```python
from build123d import *

# Parameters (mm, degrees)
SKETCH_1_W      = 5
SKETCH_1_H      = 7
SKETCH_1_H_2    = 14
SKETCH_1_W_2    = 30
SKETCH_1_H_3    = 5
EXTRUDE_2_DEPTH = 5


with BuildPart() as part:
    # 草图1 → 凸台-拉伸2 (new body)
    with BuildSketch(Plane.XY):
        with Locations((-106.5, 21.5)):
            Rectangle(SKETCH_1_W, SKETCH_1_H)
        with Locations((-111.5, 18)):
            Rectangle(SKETCH_1_W, SKETCH_1_H_2)
        Polygon((-64, 0), (-54, 0), (-54, 7), (-55.5, 7), (-55.5, 9.9), (-54, 9.9), (-54, 11), (-52, 11), (-52, 25), (-104, 25), (-104, 18), (-104, 0), (-94, 0), align=None)
        Polygon((-50, 7), (-50, 0), (-40, 0), (-10, 0), (0, 0), (0, 18), (0, 25), (-52, 25), (-52, 11), (-50, 11), (-50, 9.9), (-48.5, 9.9), (-48.5, 7), align=None)
        with Locations((7.5, 18)):
            Rectangle(SKETCH_1_W, SKETCH_1_H_2)
        with Locations((2.5, 21.5)):
            Rectangle(SKETCH_1_W, SKETCH_1_H)
        with Locations((-25, -2.5)):
            Rectangle(SKETCH_1_W_2, SKETCH_1_H_3)
        with Locations((-79, -2.5)):
            Rectangle(SKETCH_1_W_2, SKETCH_1_H_3)
    extrude(amount=EXTRUDE_2_DEPTH)


solid = part.part
```
Part model, mm, in its own coordinate system. A direction names the side the tool comes from. Round coordinates to 2 decimals unless told otherwise and drop trailing zeros. Write each loop counter-clockwise with the first axis right and the second up, starting at its lowest first coordinate (ties: lowest second). Pieces come first, ordered by that corner, then holes.
Item 1: Cut at A-A, the plane y = -3. Give the cut face in (x, z), plus the area to 3 significant figures.
Results:
outline: (-94, 0) - (-64, 0) - (-64, 5) - (-94, 5) - close; (-40, 0) - (-10, 0) - (-10, 5) - (-40, 5) - close
area: 300 mm2
Item 2: Probe L1, parallel to X at y = 16.25, z = 0.35; L2, parallel to X at y = -1.5, z = 4.45; L3, parallel to X at y = 8.25, z = 1.4. List the from-to ranges inside material, lowest first.
Results:
L1: x = -114 to -109, -104 to 0, 5 to 10
L2: x = -94 to -64, -40 to -10
L3: x = -104 to -55.5, -48.5 to 0
Item 3: Cut at B-B, the plane y = 12.25. Give the cut face in (x, z), plus the area to 3 significant figures.
Results:
outline: (-114, 0) - (-109, 0) - (-109, 5) - (-114, 5) - close; (-104, 0) - (0, 0) - (0, 5) - (-104, 5) - close; (5, 0) - (10, 0) - (10, 5) - (5, 5) - close
area: 570 mm2
Item 4: Cut at D-D, the plane y = 3.75. Give the cut face in (x, z), plus the area to 3 significant figures.
Results:
outline: (-104, 0) - (-54, 0) - (-54, 5) - (-104, 5) - close; (-50, 0) - (0, 0) - (0, 5) - (-50, 5) - close
area: 500 mm2
Item 5: Which spindle directions (+Z, -Z, +X, -X, +Y, -Y) get a long thin tool onto all of the face, cutting with end or side? Do faces 4 (the flat face through (-53, 14, 5)), 5 (the flat face through (-54, 3, 2)), 6 (the flat face through (-55.5, 8, 2)), 7 (the flat face through (-94, -3, 2)). Say none if no direction does.
Results:
face 4: +Z, +X, -X, +Y, -Y
face 5: +Z, -Z, -Y
face 6: +Z, -Z
face 7: +Z, -Z, -X, -Y
Item 6: Two-plate mould, pull along X, no slides. Class faces 1 (the flat face through (-114, 18, 2)), 2 (the flat face through (-48.5, 8, 2)), 3 (the flat face through (-99, 0, 2)): +X half, -X half, draft (parallel to the pull), parting line (faces both ways), or undercut.
Results:
face 1: -X half
face 2: undercut
face 3: draft
Item 7: Drop flat-ended pins along their axis: pin 1 Ø1 at (y, z) = (2, 1) entering from +X; pin 2 Ø1.6 at (x, z) = (-49, 3) entering from -Y; pin 3 Ø1.5 at (y, z) = (1, 3.5) entering from -X. Give the stop position or say it passes through.
Results:
pin 1: stops at x = 0
pin 2: stops at y = 0
pin 3: stops at x = -104
